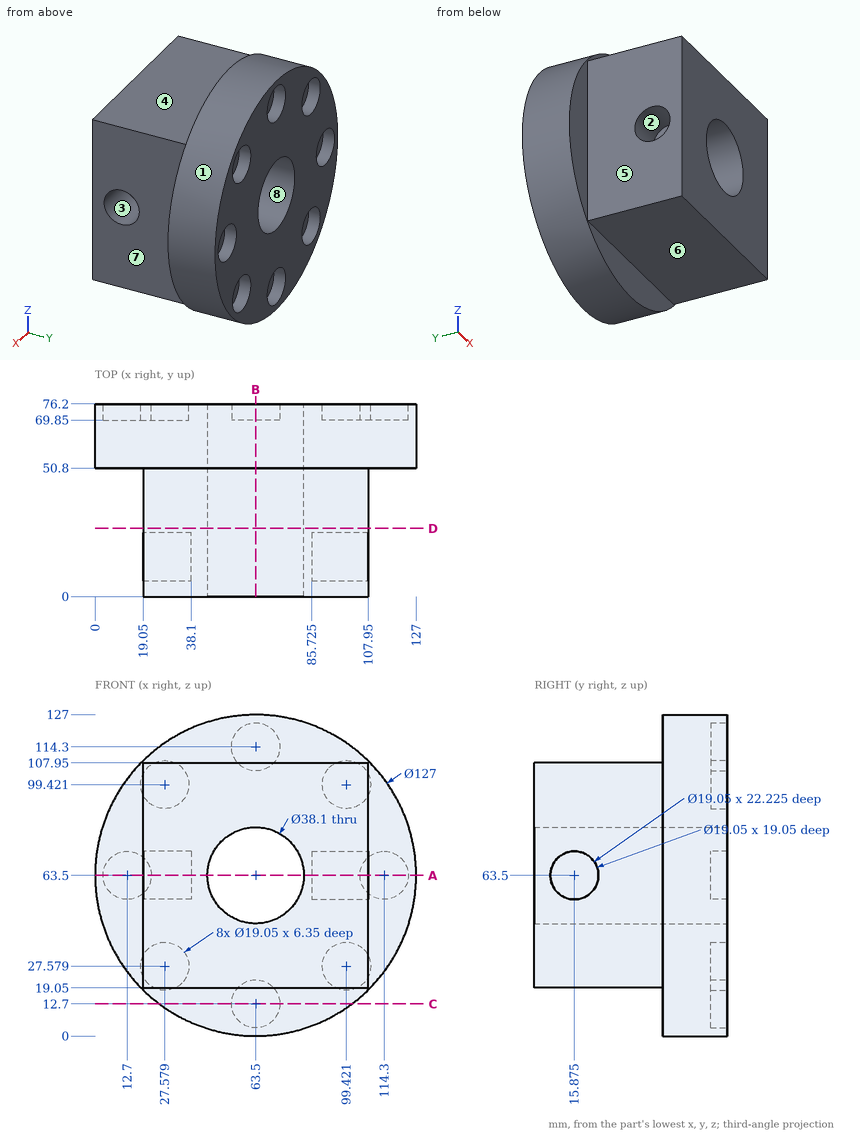
Could you check a few things on this drawing? It's one solid part, dimensions in mm from its lowest x, y, z. A direction names the side the tool comes from. Coordinates: 2 decimals unless noted, no trailing zeros. Loops run counter-clockwise (first coordinate to the right, second up) from the corner with the lowest first, then second, coordinate; pieces in that order, holes last. Notation, with made-up numbers: (25, 47) - (31, 47) arc R7 ccw to (31, 51) - close; hole circle Ø3 at (17, 72). An arc over 180 degrees is marked (long way). Answer as a JSON object with one key per item and string values. Group by question number.
Item 1: On a 3-axis mill with a long thin cutter (end or side, diameter ignored), from which of +Z, -Z, +X, -X, +Y, -Y can I reach the whole of each face in a straight line? I mean the marked faces 1, 2, 3 and 4. Say none if no direction works.
Item 2: If I drill on L1, parallel to X at y = 72, z = 63; L2, parallel to Z at x = 105.5, y = 33.5, over which ranges is the centre line in solid material (lowest first)? Write a range as from..to.
Item 3: If we section it at C-C (z = 12.7): List the corners of the cut face in (x, y) for me (3 decimals).
Item 4: If we section it at A-A (z = 63.5): List the corners of the cut face in (x, y) for me (3 decimals).
Item 5: If we section it at D-D (y = 27): List the corners of the cut face in (x, z) for me.
Item 6: For pin 1 (21 mm diameter, centred on y = 19, z = 68, fed in from +X); pin 2 (5 mm diameter, centred on x = 54, y = 48, fed in from -Z); pin 3 (12 mm diameter, centred on y = 57, z = 90, fed in from -X); pin 4 (2 mm diameter, centred on x = 54.5, z = 49, fed in from +Y), each with a flat end and sliding along its axis, tell me the tip position at first contact or that it passes through.
Item 7: If we mould it in two halves opening along X, with no side actions, what happens to the marked faces 5, 6, 7 and 8? For each: released by +X, released by -X, zero draft, split by the parting line, or undercut.
Item 8: If we section it at B-B (x = 63.5): List the corners of the cut face in (y, z) for me (3 decimals).
Returned:
{
 "1": {"face 1": "+Y, -Y", "face 2": "-X", "face 3": "+X", "face 4": "+Z, +X, -X, -Y"},
 "2": {"L1": "x = 0..3.19, 22.21..44.46, 82.54..104.79, 123.81..127", "L2": "z = 19.05..107.95"},
 "3": {"outline": "(25.4, 50.8) - (101.6, 50.8) - (101.6, 76.2) - (73.025, 76.2) - (73.025, 69.85) - (53.975, 69.85) - (53.975, 76.2) - (25.4, 76.2) - close"},
 "4": {"outline": "(0, 50.8) - (19.05, 50.8) - (19.05, 25.4) - (38.1, 25.4) - (38.1, 6.35) - (19.05, 6.35) - (19.05, 0) - (44.45, 0) - (44.45, 76.2) - (22.225, 76.2) - (22.225, 69.85) - (3.175, 69.85) - (3.175, 76.2) - (0, 76.2) - close; (82.55, 0) - (107.95, 0) - (107.95, 6.35) - (85.725, 6.35) - (85.725, 25.4) - (107.95, 25.4) - (107.95, 50.8) - (127, 50.8) - (127, 76.2) - (123.825, 76.2) - (123.825, 69.85) - (104.775, 69.85) - (104.775, 76.2) - (82.55, 76.2) - close"},
 "5": {"outline": "(19.05, 19.05) - (107.95, 19.05) - (107.95, 107.95) - (19.05, 107.95) - close; hole circle Ø38.1 at (63.5, 63.5)"},
 "6": {"pin 1": "stops at x = 107.95", "pin 2": "stops at z = 19.05", "pin 3": "stops at x = 3.4", "pin 4": "passes through"},
 "7": {"face 5": "released by -X", "face 6": "zero draft", "face 7": "released by +X", "face 8": "undercut"},
 "8": {"outline": "(0, 19.05) - (50.8, 19.05) - (50.8, 0) - (76.2, 0) - (76.2, 3.175) - (69.85, 3.175) - (69.85, 22.225) - (76.2, 22.225) - (76.2, 44.45) - (0, 44.45) - close; (0, 82.55) - (76.2, 82.55) - (76.2, 104.775) - (69.85, 104.775) - (69.85, 123.825) - (76.2, 123.825) - (76.2, 127) - (50.8, 127) - (50.8, 107.95) - (0, 107.95) - close"}
}
